The listing builds one solid part. Answer for the finished solid, in the listing's coordinates (mm). A direction names the side the tool comes from. Coordinates: 2 decimals unless noted, no trailing zeros. Loops run counter-clockwise (first coordinate to the right, second up) from the corner with the lowest first, then second, coordinate; pieces in that order, holes last. Notation, with made-up numbers: (57.25, 5) - (73.25, 5) arc R6 ccw to (73.25, 16) - close; hole circle Ø3 at (-24.75, 28). An arc over 180 degrees is marked (long way). Use one line per item in the form item = value. Start each with the question number.
```python
from build123d import *

# Parameters (mm, degrees)
F1_DEPTH      = 5
F2_T4_DEPTH   = 68.6680055615
F2_T9_DEPTH   = 69.5804590238
F2_T14_DEPTH  = 68.6556539851
F2_T19_DEPTH  = 68.6680055615
F2_T24_DEPTH  = 68.6680055615
F2_T29_DEPTH  = 68.6680055615
F2_T34_DEPTH  = 68.6680055615
F2_T39_DEPTH  = 68.6680055615
F2_T44_DEPTH  = 68.6680055615
F2_T49_DEPTH  = 68.6680055615
F2_T55_DEPTH  = 68.6680055615
F2_T59_DEPTH  = 68.6680055615
F2_T66_DEPTH  = 69.5804590238
F2_T70_DEPTH  = 68.6556539851
F2_T77_DEPTH  = 68.6680055615
F2_T81_DEPTH  = 68.6680055615
F2_T88_DEPTH  = 68.6680055615
F2_T92_DEPTH  = 68.6680055615
F2_T99_DEPTH  = 68.6680055615
F2_T103_DEPTH = 68.6680055615


# Not quite as in the source:
# - a fillet or chamfer that OpenCascade refuses, or shapes differently, is made with other operations: its cross-section is extruded or revolved along the edge and cut away or added


with BuildPart() as f1:
    # F0 (on Top) → F1 (new body)
    with BuildSketch(Plane.XY):
        Polygon((0, 0), (0, 52.987328628), (-12.5984860432, 16.3739850326), align=None)
        Polygon((12.5984860432, 17.3403284151), (0, 52.987328628), (0, 0), align=None)
        Polygon((0, 0), (-12.5984860432, 16.3739850326), (-50.3939441727, 16.3739850326), align=None)
        Polygon((50.3939441727, 16.3739850326), (12.5984860432, 17.3403284151), (0, 0), align=None)
        Polygon((20.3847786247, -6.6234160785), (0, 0), (31.1451703259, -42.8676493466), align=None)
        Polygon((0, -21.4338246733), (0, 0), (-31.1451703259, -42.8676493466), align=None)
        Polygon((-20.3847786247, -6.6234160785), (0, 0), (-50.3939441727, 16.3739850326), align=None)
        Polygon((50.3939441727, 16.3739850326), (0, 0), (20.3847786247, -6.6234160785), align=None)
        Polygon((31.1451703259, -42.8676493466), (0, 0), (0, -21.4338246733), align=None)
        Polygon((-31.1451703259, -42.8676493466), (0, 0), (-20.3847786247, -6.6234160785), align=None)
    extrude(amount=F1_DEPTH)

    # F2: chamfer of 6 on 10 edges, made by hand


with BuildPart() as f2_tool2:
    # F2_s3 → F2_t4 (new body)
    with BuildSketch(Plane(origin=(1.0926214012, -3.0915361725, 0), x_dir=(0, 0, 1), z_dir=(-0.3332244354, 0.9428475357, 0))):
        Polygon((-1, 17.6566726657), (5, 11.6566726657), (5, 17.6566726657), align=None)
    extrude(amount=F2_T4_DEPTH)

    split(bisect_by=Plane(origin=(0.451293236, 17.6509043406, 0), x_dir=(0, 0, 1), z_dir=(0.025559359, 0.9996733062, 0)), keep=Keep.TOP)


with BuildPart() as f1_1:
    add(f1.part)

    # F2_t1: cut F2_tool2
    add(f2_tool2.part, mode=Mode.SUBTRACT)


with BuildPart() as f2_tool7:
    # F2_s8 → F2_t9 (new body)
    with BuildSketch(Plane(origin=(21.3229816345, 61.9682119253, 0), x_dir=(0, 0, 1), z_dir=(-0.3253719116, -0.9455861247, 0))):
        Polygon((-1, 17.2405884042), (5, 11.2405884042), (5, 17.2405884042), align=None)
    extrude(amount=F2_T9_DEPTH)

    split(bisect_by=Plane.XZ.offset(-16.3739850326), keep=Keep.BOTTOM)


with BuildPart() as f1_2:
    add(f1_1.part)

    # F2_t6: cut F2_tool7
    add(f2_tool7.part, mode=Mode.SUBTRACT)


with BuildPart() as f2_tool12:
    # F2_s13 → F2_t14 (new body)
    with BuildSketch(Plane.YZ.offset(2.8316118846)):
        Polygon((16.3739850326, -1), (10.3739850326, 5), (16.3739850326, 5), align=None)
    extrude(amount=-F2_T14_DEPTH)

    split(bisect_by=Plane(origin=(-16.3024611761, 5.6096032055, 0), x_dir=(0, 0, 1), z_dir=(-0.9455861247, 0.3253719116, 0)), keep=Keep.TOP)


with BuildPart() as f1_3:
    add(f1_2.part)

    # F2_t11: cut F2_tool12
    add(f2_tool12.part, mode=Mode.SUBTRACT)


with BuildPart() as f2_tool17:
    # F2_s18 → F2_t19 (new body)
    with BuildSketch(Plane(origin=(-51.9012195214, 39.7742870116, 0), x_dir=(0, 0, 1), z_dir=(0.7937292793, -0.6082711823, 0))):
        Polygon((-1, 17.6566726657), (5, 11.6566726657), (5, 17.6566726657), align=None)
    extrude(amount=F2_T19_DEPTH)

    split(bisect_by=Plane(origin=(-16.926464871, 5.0252240345, 0), x_dir=(0, 0, 1), z_dir=(-0.9586440884, 0.2846076455, 0)), keep=Keep.TOP)


with BuildPart() as f1_4:
    add(f1_3.part)

    # F2_t16: cut F2_tool17
    add(f2_tool17.part, mode=Mode.SUBTRACT)


with BuildPart() as f2_tool22:
    # F2_s23 → F2_t24 (new body)
    with BuildSketch(Plane(origin=(0.9332100871, 3.1433320482, 0), x_dir=(0, 0, 1), z_dir=(-0.2846076455, -0.9586440884, 0))):
        Polygon((-1, 17.6566726657), (5, 11.6566726657), (5, 17.6566726657), align=None)
    extrude(amount=F2_T24_DEPTH)

    split(bisect_by=Plane(origin=(-10.7400451584, -14.014618069, 0), x_dir=(0, 0, 1), z_dir=(-0.6082711823, -0.7937292793, 0)), keep=Keep.TOP)


with BuildPart() as f1_5:
    add(f1_4.part)

    # F2_t21: cut F2_tool22
    add(f2_tool22.part, mode=Mode.SUBTRACT)


with BuildPart() as f2_tool27:
    # F2_s28 → F2_t29 (new body)
    with BuildSketch(Plane(origin=(-53.8659537043, -37.0700624038, 0), x_dir=(0, 0, 1), z_dir=(0.8237761079, 0.5669152707, 0))):
        Polygon((-1, 17.6566726657), (5, 11.6566726657), (5, 17.6566726657), align=None)
    extrude(amount=F2_T29_DEPTH)

    split(bisect_by=Plane(origin=(-10.0098373636, -14.5451450862, 0), x_dir=(0, 0, 1), z_dir=(-0.5669152707, -0.8237761079, 0)), keep=Keep.TOP)


with BuildPart() as f1_6:
    add(f1_5.part)

    # F2_t26: cut F2_tool27
    add(f2_tool27.part, mode=Mode.SUBTRACT)


with BuildPart() as f2_tool32:
    # F2_s33 → F2_t34 (new body)
    with BuildSketch(Plane(origin=(-2.7011086511, 1.8588785563, 0), x_dir=(0, 0, 1), z_dir=(0.8237761079, -0.5669152707, 0))):
        Polygon((-1, 17.6566726657), (5, 11.6566726657), (5, 17.6566726657), align=None)
    extrude(amount=F2_T34_DEPTH)

    split(bisect_by=Plane(origin=(10.0098373636, -14.5451450862, 0), x_dir=(0, 0, 1), z_dir=(0.5669152707, -0.8237761079, 0)), keep=Keep.TOP)


with BuildPart() as f1_7:
    add(f1_6.part)

    # F2_t31: cut F2_tool32
    add(f2_tool32.part, mode=Mode.SUBTRACT)


with BuildPart() as f2_tool37:
    # F2_s38 → F2_t39 (new body)
    with BuildSketch(Plane(origin=(18.6102292957, -62.6848455422, 0), x_dir=(0, 0, 1), z_dir=(-0.2846076455, 0.9586440884, 0))):
        Polygon((-1, 17.6566726657), (5, 11.6566726657), (5, 17.6566726657), align=None)
    extrude(amount=F2_T39_DEPTH)

    split(bisect_by=Plane(origin=(10.7400451584, -14.014618069, 0), x_dir=(0, 0, 1), z_dir=(0.6082711823, -0.7937292793, 0)), keep=Keep.TOP)


with BuildPart() as f1_8:
    add(f1_7.part)

    # F2_t36: cut F2_tool37
    add(f2_tool37.part, mode=Mode.SUBTRACT)


with BuildPart() as f2_tool42:
    # F2_s43 → F2_t44 (new body)
    with BuildSketch(Plane(origin=(-2.6025870408, -1.9944819195, 0), x_dir=(0, 0, 1), z_dir=(0.7937292793, 0.6082711823, 0))):
        Polygon((-1, 17.6566726657), (5, 11.6566726657), (5, 17.6566726657), align=None)
    extrude(amount=F2_T44_DEPTH)

    split(bisect_by=Plane(origin=(16.926464871, 5.0252240345, 0), x_dir=(0, 0, 1), z_dir=(0.9586440884, 0.2846076455, 0)), keep=Keep.TOP)


with BuildPart() as f1_9:
    add(f1_8.part)

    # F2_t41: cut F2_tool42
    add(f2_tool42.part, mode=Mode.SUBTRACT)


with BuildPart() as f2_tool47:
    # F2_s48 → F2_t49 (new body)
    with BuildSketch(Plane(origin=(65.3677079475, -1.6713027209, 0), x_dir=(0, 0, 1), z_dir=(-0.9996733062, 0.025559359, 0))):
        Polygon((-1, 17.6566726657), (5, 11.6566726657), (5, 17.6566726657), align=None)
    extrude(amount=F2_T49_DEPTH)

    split(bisect_by=Plane(origin=(16.6475503122, 5.8836347802, 0), x_dir=(0, 0, 1), z_dir=(0.9428475357, 0.3332244354, 0)), keep=Keep.TOP)


with BuildPart() as f1_10:
    add(f1_9.part)

    # F2_t46: cut F2_tool47
    add(f2_tool47.part, mode=Mode.SUBTRACT)


with BuildPart() as f2_tool53:
    # F2_s54 → F2_t55 (new body)
    with BuildSketch(Plane(origin=(1.0926214012, -3.0915361725, 0), x_dir=(0, 0, 1), z_dir=(-0.3332244354, 0.9428475357, 0))):
        Polygon((-1, 17.6566726657), (5, 11.6566726657), (5, 17.6566726657), align=None)
    extrude(amount=F2_T55_DEPTH)

    split(bisect_by=Plane(origin=(0.451293236, 17.6509043406, 0), x_dir=(0, 0, 1), z_dir=(-0.025559359, -0.9996733062, 0)), keep=Keep.TOP)


with BuildPart() as f2_tool57:
    # F2_s58 → F2_t59 (new body)
    with BuildSketch(Plane(origin=(65.3677079475, -1.6713027209, 0), x_dir=(0, 0, 1), z_dir=(-0.9996733062, 0.025559359, 0))):
        Polygon((-1, 17.6566726657), (5, 11.6566726657), (5, 17.6566726657), align=None)
    extrude(amount=F2_T59_DEPTH)

    split(bisect_by=Plane(origin=(16.6475503122, 5.8836347802, 0), x_dir=(0, 0, 1), z_dir=(-0.9428475357, -0.3332244354, 0)), keep=Keep.TOP)


with BuildPart() as f2_tool53_1:
    add(f2_tool53.part)

    # F2_t61: intersect F2_tool57
    add(f2_tool57.part, mode=Mode.INTERSECT)


with BuildPart() as f1_11:
    add(f1_10.part)

    # F2_t51: cut F2_tool53
    add(f2_tool53_1.part, mode=Mode.SUBTRACT)


with BuildPart() as f2_tool64:
    # F2_s65 → F2_t66 (new body)
    with BuildSketch(Plane(origin=(21.3229816345, 61.9682119253, 0), x_dir=(0, 0, 1), z_dir=(-0.3253719116, -0.9455861247, 0))):
        Polygon((-1, 17.2405884042), (5, 11.2405884042), (5, 17.2405884042), align=None)
    extrude(amount=F2_T66_DEPTH)

    split(bisect_by=Plane.XZ.offset(-16.3739850326), keep=Keep.TOP)


with BuildPart() as f2_tool68:
    # F2_s69 → F2_t70 (new body)
    with BuildSketch(Plane.YZ.offset(2.8316118846)):
        Polygon((16.3739850326, -1), (10.3739850326, 5), (16.3739850326, 5), align=None)
    extrude(amount=-F2_T70_DEPTH)

    split(bisect_by=Plane(origin=(-16.3024611761, 5.6096032055, 0), x_dir=(0, 0, 1), z_dir=(0.9455861247, -0.3253719116, 0)), keep=Keep.TOP)


with BuildPart() as f2_tool64_1:
    add(f2_tool64.part)

    # F2_t72: intersect F2_tool68
    add(f2_tool68.part, mode=Mode.INTERSECT)


with BuildPart() as f1_12:
    add(f1_11.part)

    # F2_t62: cut F2_tool64
    add(f2_tool64_1.part, mode=Mode.SUBTRACT)


with BuildPart() as f2_tool75:
    # F2_s76 → F2_t77 (new body)
    with BuildSketch(Plane(origin=(-51.9012195214, 39.7742870116, 0), x_dir=(0, 0, 1), z_dir=(0.7937292793, -0.6082711823, 0))):
        Polygon((-1, 17.6566726657), (5, 11.6566726657), (5, 17.6566726657), align=None)
    extrude(amount=F2_T77_DEPTH)

    split(bisect_by=Plane(origin=(-16.926464871, 5.0252240345, 0), x_dir=(0, 0, 1), z_dir=(0.9586440884, -0.2846076455, 0)), keep=Keep.TOP)


with BuildPart() as f2_tool79:
    # F2_s80 → F2_t81 (new body)
    with BuildSketch(Plane(origin=(0.9332100871, 3.1433320482, 0), x_dir=(0, 0, 1), z_dir=(-0.2846076455, -0.9586440884, 0))):
        Polygon((-1, 17.6566726657), (5, 11.6566726657), (5, 17.6566726657), align=None)
    extrude(amount=F2_T81_DEPTH)

    split(bisect_by=Plane(origin=(-10.7400451584, -14.014618069, 0), x_dir=(0, 0, 1), z_dir=(0.6082711823, 0.7937292793, 0)), keep=Keep.TOP)


with BuildPart() as f2_tool75_1:
    add(f2_tool75.part)

    # F2_t83: intersect F2_tool79
    add(f2_tool79.part, mode=Mode.INTERSECT)


with BuildPart() as f1_13:
    add(f1_12.part)

    # F2_t73: cut F2_tool75
    add(f2_tool75_1.part, mode=Mode.SUBTRACT)


with BuildPart() as f2_tool86:
    # F2_s87 → F2_t88 (new body)
    with BuildSketch(Plane(origin=(-53.8659537043, -37.0700624038, 0), x_dir=(0, 0, 1), z_dir=(0.8237761079, 0.5669152707, 0))):
        Polygon((-1, 17.6566726657), (5, 11.6566726657), (5, 17.6566726657), align=None)
    extrude(amount=F2_T88_DEPTH)

    split(bisect_by=Plane(origin=(-10.0098373636, -14.5451450862, 0), x_dir=(0, 0, 1), z_dir=(0.5669152707, 0.8237761079, 0)), keep=Keep.TOP)


with BuildPart() as f2_tool90:
    # F2_s91 → F2_t92 (new body)
    with BuildSketch(Plane(origin=(-2.7011086511, 1.8588785563, 0), x_dir=(0, 0, 1), z_dir=(0.8237761079, -0.5669152707, 0))):
        Polygon((-1, 17.6566726657), (5, 11.6566726657), (5, 17.6566726657), align=None)
    extrude(amount=F2_T92_DEPTH)

    split(bisect_by=Plane(origin=(10.0098373636, -14.5451450862, 0), x_dir=(0, 0, 1), z_dir=(-0.5669152707, 0.8237761079, 0)), keep=Keep.TOP)


with BuildPart() as f2_tool86_1:
    add(f2_tool86.part)

    # F2_t94: intersect F2_tool90
    add(f2_tool90.part, mode=Mode.INTERSECT)


with BuildPart() as f1_14:
    add(f1_13.part)

    # F2_t84: cut F2_tool86
    add(f2_tool86_1.part, mode=Mode.SUBTRACT)


with BuildPart() as f2_tool97:
    # F2_s98 → F2_t99 (new body)
    with BuildSketch(Plane(origin=(18.6102292957, -62.6848455422, 0), x_dir=(0, 0, 1), z_dir=(-0.2846076455, 0.9586440884, 0))):
        Polygon((-1, 17.6566726657), (5, 11.6566726657), (5, 17.6566726657), align=None)
    extrude(amount=F2_T99_DEPTH)

    split(bisect_by=Plane(origin=(10.7400451584, -14.014618069, 0), x_dir=(0, 0, 1), z_dir=(-0.6082711823, 0.7937292793, 0)), keep=Keep.TOP)


with BuildPart() as f2_tool101:
    # F2_s102 → F2_t103 (new body)
    with BuildSketch(Plane(origin=(-2.6025870408, -1.9944819195, 0), x_dir=(0, 0, 1), z_dir=(0.7937292793, 0.6082711823, 0))):
        Polygon((-1, 17.6566726657), (5, 11.6566726657), (5, 17.6566726657), align=None)
    extrude(amount=F2_T103_DEPTH)

    split(bisect_by=Plane(origin=(16.926464871, 5.0252240345, 0), x_dir=(0, 0, 1), z_dir=(-0.9586440884, -0.2846076455, 0)), keep=Keep.TOP)


with BuildPart() as f2_tool97_1:
    add(f2_tool97.part)

    # F2_t105: intersect F2_tool101
    add(f2_tool101.part, mode=Mode.INTERSECT)


with BuildPart() as f1_15:
    add(f1_14.part)

    # F2_t95: cut F2_tool97
    add(f2_tool97_1.part, mode=Mode.SUBTRACT)


solid = f1_15.part
```
(1) Determine the mould class of faces 1 (the face through (30.303, 5.343, 2.465)), 2 (the face through (-21.375, -22.134, 2.465)), 3 (the face through (-11.317, -25.016, 2.465)) for opening direction X: +X half, -X half, draft (parallel to the pull), parting line (faces both ways), or undercut.
(2) Find the intervals of material crossed by probe 1 along X at (y, z) = (-20, 4.55); probe 2 along X at (y, z) = (-31, 1.1); probe 3 along Y at (x, z) = (33.5, 4.35), in increasing order. Write a range as from..to.
(3) A cutting plane is placed at B-B (z = 2.9). Determine the outline of the cut face in (x, y), then the cut area to 3 significant figures.
(4) A cutting plane is placed at A-A (y = -22). Determine the outline of the cut face in (x, z).
(5) A cutting plane is placed at D-D (y = 13). Determine the outline of the cut face in (x, z).
(6) A cutting plane is placed at C-C (x = -10). Determine the outline of the cut face in (y, z), then the cut area to 3 significant figures.
(7) For faces 4 (the face through (-27.608, 12.909, 2.465)), 5 (the face through (14.445, -27.169, 2.465)), 6 (the face through (-27.25, 3, 2.46)), determine the directions among +Z, -Z, +X, -X, +Y, -Y from which every point of the face is accessible in a straight line to the end or side of a thin tool.
(8) Each of these flat-tipped pins is pushed along its axis until it touches: pin 1 Ø1 at (x, z) = (-34.5, 1) entering from -Y; pin 2 Ø3 at (x, z) = (34, 3) entering from -Y; pin 3 Ø3 at (x, z) = (2, 2) entering from -Y. Where does it stop, or does it pass through?
Evaluation:
q1.face_1 = +X half
q1.face_2 = -X half
q1.face_3 = undercut
q2.probe_1 = -18.57..-7.71, 7.71..18.57
q2.probe_2 = -25.43..-17.6, 17.6..25.43
q2.probe_3 = 10.17..11.45
q3.outline = (-38.89, 12.47) - (-15.88, -5.16) - (-24.27, -33.4) - (0, -16.7) - (24.27, -33.4) - (15.88, -5.16) - (39.26, 12.76) - (9.82, 13.51) - (0.05, 41.14) - (-9.82, 12.47) - close
q3.area = 2,000 mm^2
q4.outline = (-23.91, 0) - (-2.59, 0) - (-11.41, 5) - (-18.69, 5) - close; (2.59, 0) - (23.91, 0) - (18.69, 5) - (11.41, 5) - close
q5.outline = (-44.35, 0) - (44.35, 0) - (40.01, 2.64) - (9.45, 3.42) - (7.77, 5) - (-7.41, 5) - (-10.19, 2.37) - (-40.44, 2.37) - close
q6.outline = (-27.1, 0) - (20.85, 0) - (12.73, 2.64) - (10.37, 5) - (-21.03, 5) - close
q6.area = 192 mm^2
q7.face_4 = +Z, -X, +Y
q7.face_5 = +Z, -Y
q7.face_6 = +Z, -X
q8.pin_1 = 5.98
q8.pin_2 = 6.64
q8.pin_3 = -21.26
